Here's how the part is built. I have some questions about the finished solid (model axes, mm). A direction names the side the tool comes from. Coordinates: 2 decimals unless noted, no trailing zeros. Order: outer loops, then holes, each group sorted by start corner. A loop starts at its lowest first (then second) coordinate and runs counter-clockwise, first axis right, second up. Notation, with made-up numbers: (23, 63.5) - (67, 63.5) arc R29 ccw to (67, 100.5) - close; hole circle Ø1 at (53.5, -4.75). An arc over 180 degrees is marked (long way). Use one line per item in the form item = value. Start each with the question number.
from build123d import *

# Parameters (mm, degrees)
CUT_EXTRUDE_START        = -6.062177826
CUT_EXTRUDE_1_OUTLINE_W  = 4.5
CUT_EXTRUDE_1_OUTLINE_H  = 16
CUT_EXTRUDE_1_DEPTH      = 12.124355652
CUT_EXTRUDE_2_DEPTH      = 15.43086969
CUT_EXTRUDE_2_DEPTH_BACK = 15.43086969
SKETCH_3_R               = 2
SKETCH_4_W               = 7.475945476
SKETCH_4_H               = 17.759961534
EXTRUDE_1_DEPTH          = 7
SKETCH_5_R               = 2
CUT_EXTRUDE_3_DEPTH      = 15


# Read off the part's stored shape, not the designer's step: 切除-拉伸1
with BuildPart() as part:
    # 草图1 → 旋转1 (revolve)
    with BuildSketch(Plane(origin=(0, 0, 0), x_dir=(0, 0, -1), z_dir=(1, 0, 0))):
        with BuildLine():
            Line((0, 7), (0, -7))
            ThreePointArc((0, -7), (-7, 0), (0, 7))
        make_face()
    revolve(axis=Axis((0, 7, 0), (0, -1, 0)))

    # 切除-拉伸1 outline → 切除-拉伸1 (cut)
    with BuildSketch(Plane.XY.offset(CUT_EXTRUDE_START)):
        with Locations((-5.75, 0)):
            Rectangle(CUT_EXTRUDE_1_OUTLINE_W, CUT_EXTRUDE_1_OUTLINE_H)
        with Locations((5.75, 0)):
            Rectangle(CUT_EXTRUDE_1_OUTLINE_W, CUT_EXTRUDE_1_OUTLINE_H)
    extrude(amount=CUT_EXTRUDE_1_DEPTH, mode=Mode.SUBTRACT)

    # 草图3 → 切除-拉伸2 (cut, two sides: drawn at the far end of the back side and taken through both)
    with BuildSketch(Plane(origin=(3.5, 0, 0), x_dir=(0, 0, -1), z_dir=(1, 0, 0)).offset(-CUT_EXTRUDE_2_DEPTH_BACK)):
        Circle(SKETCH_3_R)
    extrude(amount=CUT_EXTRUDE_2_DEPTH + CUT_EXTRUDE_2_DEPTH_BACK, mode=Mode.SUBTRACT)

    # 草图4 → 凸台-拉伸1 (add)
    with BuildSketch(Plane(origin=(3.5, 0, 0), x_dir=(0, 0, -1), z_dir=(1, 0, 0))):
        with Locations((0, -13.120019233)):
            Rectangle(SKETCH_4_W, SKETCH_4_H)
    extrude(amount=-EXTRUDE_1_DEPTH)

    # 草图5 → 切除-拉伸3 (cut)
    with BuildSketch(Plane.XZ.offset(22)):
        with Locations(Location((0, 0, 0), (0, 0, 270))):
            Circle(SKETCH_5_R)
    extrude(amount=-CUT_EXTRUDE_3_DEPTH, mode=Mode.SUBTRACT)


solid = part.part
1) For pin 1 (2 mm diameter, centred on x = 2, y = 2.5, fed in from +Z); pin 2 (3.5 mm diameter, centred on x = 1.5, y = -17.5, fed in from -Z); pin 3 (1.5 mm diameter, centred on x = 0.5, y = -2, fed in from +Z), each with a flat end and sliding along its axis, tell me the tip position at first contact or that it passes through.
2) Suppose I cut it at C-C, the plane y = 1. List the corners of the cut face in (x, z) for me.
3) Suppose I cut it at D-D, the plane y = -13.5. List the corners of the cut face in (x, z) for me.
4) Suppose I cut it at B-B, the plane x = 0. List the corners of the cut face in (y, z) for me, then the cut area to 3 significant figures.
5) If we mould it in two halves opening along Z, with no side actions, what happens to faces 3 (the flat face through (-3.5, -8, 0)), 4 (the flat face through (0, -14, 3.738)), 5 (the cylindrical face through (0, -2, 0)), 6 (the cylindrical face through (-2, -15, 0))? For each: pulls with the +Z half, pulls with the -Z half, needs draft (parallel to the pull), parting line crosses it, or undercut.
6) I need wall thicknesses on probe 1 along X at (y, z) = (-13, 0); probe 2 along Z at (x, y) = (-3, -6); probe 3 along Z at (x, y) = (0.5, -8). Which ranges of each line are inside material? Lowest first, please. Write a range as [from, to].
7) Which directions (+Z, -Z, +X, -X, +Y, -Y) give clear straight access to the entire face, cutting with the end or side of a thin tool? Please do faces 1 (the flat face through (3.5, -8, 0)), 2 (the flat face through (0, -7, 0)).
8) Suppose I cut it at A-A, the plane z = -1.5. List the corners of the cut face in (x, y) for me.
From the geometry:
q1.pin_1 = 6.64
q1.pin_2 = -3.74
q1.pin_3 = 6.88
q2.outline = (-3.5, -5.98) arc R6.93 ccw to (3.5, -5.98) - (3.5, -1.73) - (-3.5, -1.73) - close; (-3.5, 1.73) - (3.5, 1.73) - (3.5, 5.98) arc R6.93 ccw to (-3.5, 5.98) - close
q3.outline = (-3.5, -3.74) - (3.5, -3.74) - (3.5, 3.74) - (-3.5, 3.74) - close; hole circle Ø4 at (0, 0)
q4.outline = (-22, -3.74) - (-5.92, -3.74) arc R7 ccw (long way) to (-5.92, 3.74) - (-22, 3.74) - (-22, 2) - (-7, 2) - (-7, -2) - (-22, -2) - close; hole circle Ø4 at (0, 0)
q4.area = 196 mm2
q5.face_3 = needs draft
q5.face_4 = pulls with the +Z half
q5.face_5 = undercut
q5.face_6 = undercut
q6.probe_1 = [-3.5, -2], [2, 3.5]
q6.probe_2 = [-3.74, 3.74]
q6.probe_3 = [-3.74, -1.94], [1.94, 3.74]
q7.face_1 = +Z, -Z, +X, +Y, -Y
q7.face_2 = -Y
q8.outline = (-3.5, -22) - (-1.32, -22) - (-1.32, -7) - (1.32, -7) - (1.32, -22) - (3.5, -22) - (3.5, -1.32) - (-3.5, -1.32) - close; (-3.5, 1.32) - (3.5, 1.32) - (3.5, 5.87) arc R6.84 ccw to (-3.5, 5.87) - close
